```python
from build123d import *

# Parameters (mm, degrees)
SKETCH_1_W          = 6
SKETCH_1_H          = 60
EXTRUDE_1_DEPTH     = 20
SKETCH_2_W          = 5
SKETCH_2_H          = 30
EXTRUDE_2_DEPTH     = 8
SKETCH_3_W          = 10
SKETCH_3_H          = 30
EXTRUDE_3_DEPTH     = 2
SKETCH_4_W          = 1.5
SKETCH_4_H          = 1.5
EXTRUDE_4_DEPTH     = 30
SKETCH_6_W          = 20
SKETCH_6_H          = 15
EXTRUDE_5_DEPTH     = 3
SKETCH_7_R          = 5
CUT_EXTRUDE_1_DEPTH = 42.448763552
SKETCH_8_R          = 7.5
SKETCH_8_R_2        = 5
SKETCH_8_R_3        = 7.459139247
EXTRUDE_7_DEPTH     = 3
CUT_EXTRUDE_START   = -1
SKETCH_10_R         = 5
CUT_EXTRUDE_3_DEPTH = 1
SKETCH_11_W         = 26
SKETCH_11_H         = 15
EXTRUDE_8_DEPTH     = 3
SKETCH_12_R         = 5
CUT_EXTRUDE_4_DEPTH = 3


with BuildPart() as part:
    # 草图1 → 凸台-拉伸1 (new body)
    with BuildSketch(Plane.XY):
        Rectangle(SKETCH_1_W, SKETCH_1_H)
    extrude(amount=EXTRUDE_1_DEPTH)

    # 草图2 → 凸台-拉伸2 (add)
    with BuildSketch(Plane(origin=(3, 0, 0), x_dir=(0, 0, -1), z_dir=(1, 0, 0))):
        with Locations((-17.5, 0)):
            Rectangle(SKETCH_2_W, SKETCH_2_H)
        with Locations((-2.5, 0)):
            Rectangle(SKETCH_2_W, SKETCH_2_H)
    extrude(amount=EXTRUDE_2_DEPTH)

    # 草图3 → 凸台-拉伸3 (add)
    with BuildSketch(Plane(origin=(3, 0, 0), x_dir=(0, 0, -1), z_dir=(1, 0, 0))):
        with Locations((-10, 0)):
            Rectangle(SKETCH_3_W, SKETCH_3_H)
    extrude(amount=EXTRUDE_3_DEPTH)

    # 草图4 → 凸台-拉伸4 (add)
    with BuildSketch(Plane.XZ.offset(15)):
        with Locations((7.75, 14.25)):
            Rectangle(SKETCH_4_W, SKETCH_4_H)
        with Locations((7.75, 5.75)):
            Rectangle(SKETCH_4_W, SKETCH_4_H)
    extrude(amount=-EXTRUDE_4_DEPTH)

    # 草图6 → 凸台-拉伸5 (add)
    with BuildSketch(Plane(origin=(0, 0, 0), x_dir=(-1, 0, 0), z_dir=(0, 0, -1))):
        with Locations((13, 22.5)):
            Rectangle(SKETCH_6_W, SKETCH_6_H)
        with Locations((13, -22.5)):
            Rectangle(SKETCH_6_W, SKETCH_6_H)
    extrude(amount=-EXTRUDE_5_DEPTH)

    # 草图7 → 切除-拉伸1 (cut, through all)
    with BuildSketch(Plane.XY.offset(3)):
        with Locations((-13, -22.5)):
            Circle(SKETCH_7_R)
        with Locations((-13, 22.5)):
            Circle(SKETCH_7_R)
    extrude(amount=-CUT_EXTRUDE_1_DEPTH, mode=Mode.SUBTRACT)

    # 草图8 → 凸台-拉伸7 (add)
    # profile 1 of 4: a face of its own
    with BuildSketch(Plane.ZY.offset(3)):
        with Locations((12.5, 22.5)):
            Circle(SKETCH_8_R)
        with Locations((12.5, 22.5)):
            Circle(SKETCH_8_R_2, mode=Mode.SUBTRACT)
    # profile 2 of 4: a face of its own
    with BuildSketch(Plane.ZY.offset(3)):
        with BuildLine():
            Line((12.5, 30), (3, 30))
            Line((3, 30), (3, 15))
            Line((3, 15), (12.5, 15))
            ThreePointArc((12.5, 15), (5, 22.5), (12.5, 30))
        make_face()
    # profile 3 of 4: a face of its own
    with BuildSketch(Plane.ZY.offset(3)):
        with BuildLine():
            Line((12.540860753, -15.081721505), (3, -15.081721505))
            Line((3, -15.081721505), (3, -30))
            Line((3, -30), (12.540860753, -30))
            ThreePointArc((12.540860753, -30), (5.081721505, -22.540860753), (12.540860753, -15.081721505))
        make_face()
    # profile 4 of 4: a face of its own
    with BuildSketch(Plane.ZY.offset(3)):
        with Locations((12.540860753, -22.540860753)):
            Circle(SKETCH_8_R_3)
        with Locations((12.540860753, -22.540860753)):
            Circle(SKETCH_8_R_2, mode=Mode.SUBTRACT)
    extrude(amount=EXTRUDE_7_DEPTH)

    # 草图10 → 切除-拉伸3 (cut)
    with BuildSketch(Plane.ZY.offset(3).offset(CUT_EXTRUDE_START)):
        with Locations((12.5, 22.5)):
            Circle(SKETCH_10_R)
        with Locations((12.540860753, -22.540860753)):
            Circle(SKETCH_10_R)
    extrude(amount=CUT_EXTRUDE_3_DEPTH, mode=Mode.SUBTRACT)

    # 草图11 → 凸台-拉伸8 (add)
    with BuildSketch(Plane(origin=(0, 0, 0), x_dir=(-1, 0, 0), z_dir=(0, 0, -1))):
        with Locations((10, 22.5)):
            Rectangle(SKETCH_11_W, SKETCH_11_H)
        with Locations((10, -22.5)):
            Rectangle(SKETCH_11_W, SKETCH_11_H)
    extrude(amount=EXTRUDE_8_DEPTH)

    # 草图12 → 切除-拉伸4 (cut)
    with BuildSketch(Plane.XY):
        with Locations((-13, 22.5)):
            Circle(SKETCH_12_R)
        with Locations((-13, -22.5)):
            Circle(SKETCH_12_R)
    extrude(amount=-CUT_EXTRUDE_4_DEPTH, mode=Mode.SUBTRACT)


solid = part.part
```
Could you check a few things on this model? Use its own coordinates, in mm. A direction names the side the tool comes from. Give positions to 0.01 mm unless a question says otherwise; leave off trailing zeros. Loops run counter-clockwise (first coordinate to the right, second up) from the corner with the lowest first, then second, coordinate; pieces in that order, holes last. Notation, with made-up numbers: (44, 18.5) - (69, 18.5) arc R29 ccw to (69, 54.5) - close; hole circle Ø10 at (-14, 33). An arc over 180 degrees is marked (long way). Answer in a Markdown table with one row per item. Add a question column.
Q1. If we section it at B-B (x = -12.5): List the corners of the cut face in (y, z) for me, plus the area to 3 significant figures.
Q2. If we section it at C-C (y = 2.5): List the corners of the cut face in (x, z) for me.
Q3. Please list where these lines run through material, in increasing order: L1, parallel to Y at x = -13, z = 1.5; L2, parallel to Y at x = -14, z = 1.5; L3, parallel to X at y = 27, z = 14.25. Write a range as from..to.
Q4. Which directions (+Z, -Z, +X, -X, +Y, -Y) give clear straight access to the entire face, cutting with the end or side of a thin tool? Please do faces 4 (the face through (-4.48, 22.34, 20)), 5 (the face through (-6, 24.3, 7.6)), 6 (the face through (3, 22, 9)), 7 (the face through (6, 0, 5)).
Q5. If we section it at A-A (z = 1.75): List the corners of the cut face in (x, y) for me, plus the area to 3 significant figures.
Q6. We'd pull the mould along X, two halves only. Please class faces 1 (the face through (11, 0, 3)), 2 (the face through (4, 15, 10)), 3 (the face through (5, 0, 10)): +X half, -X half, draft (parallel to the pull), parting line (faces both ways), or undercut.
Q7. For pin 1 (9 mm diameter, centred on y = -22.54, z = 12.54, fed in from +X); pin 2 (8 mm diameter, centred on y = -26, z = 17, fed in from -X); pin 3 (8 mm diameter, centred on y = 22.5, z = 12.5, fed in from -X), each with a flat end and sliding along its axis, tell me the tip position at first contact or that it passes through.
Q8. If we section it at D-D (y = 19): List the corners of the cut face in (x, z) for me.
The answers:
| question | item | result |
|---|---|---|
| 1 | outline | (-30, -3) - (-27.47, -3) - (-27.47, 3) - (-30, 3) - close; (-17.53, -3) - (-15, -3) - (-15, 3) - (-17.53, 3) - close; (15, -3) - (17.53, -3) - (17.53, 3) - (15, 3) - close; (27.47, -3) - (30, -3) - (30, 3) - (27.47, 3) - close |
| 1 | area | 60.6 mm^2 |
| 2 | outline | (-3, 0) - (11, 0) - (11, 5) - (8.5, 5) - (8.5, 6.5) - (7, 6.5) - (7, 5) - (5, 5) - (5, 15) - (7, 15) - (7, 13.5) - (8.5, 13.5) - (8.5, 15) - (11, 15) - (11, 20) - (-3, 20) - close |
| 3 | L1 | y = -30..-27.5, -17.5..-15, 15..17.5, 27.5..30 |
| 3 | L2 | y = -30..-27.4, -17.6..-15, 15..17.6, 27.4..30 |
| 3 | L3 | x = -2..3 |
| 4 | face 4 | +Z, -X |
| 4 | face 5 | +Z, -X, +Y, -Y |
| 4 | face 6 | +Z, -Z, +X, +Y |
| 4 | face 7 | +Y, -Y |
| 5 | outline | (-23, -30) - (3, -30) - (3, -15) - (11, -15) - (11, 15) - (3, 15) - (3, 30) - (-23, 30) - (-23, 15) - (-3, 15) - (-3, -15) - (-23, -15) - close; hole circle Ø10 at (-13, -22.5); hole circle Ø10 at (-13, 22.5) |
| 5 | area | 1,040 mm^2 |
| 6 | face 1 | +X half |
| 6 | face 2 | draft |
| 6 | face 3 | undercut |
| 7 | pin 1 | stops at x = 3 |
| 7 | pin 2 | stops at x = -6 |
| 7 | pin 3 | stops at x = -2 |
| 8 | outline | (-23, -3) - (-16.57, -3) - (-16.57, 3) - (-23, 3) - close; (-9.43, -3) - (3, -3) - (3, 20) - (-3, 20) - (-3, 19.13) - (-6, 19.13) - (-6, 16.07) - (-2, 16.07) - (-2, 8.93) - (-6, 8.93) - (-6, 3) - (-9.43, 3) - close |
